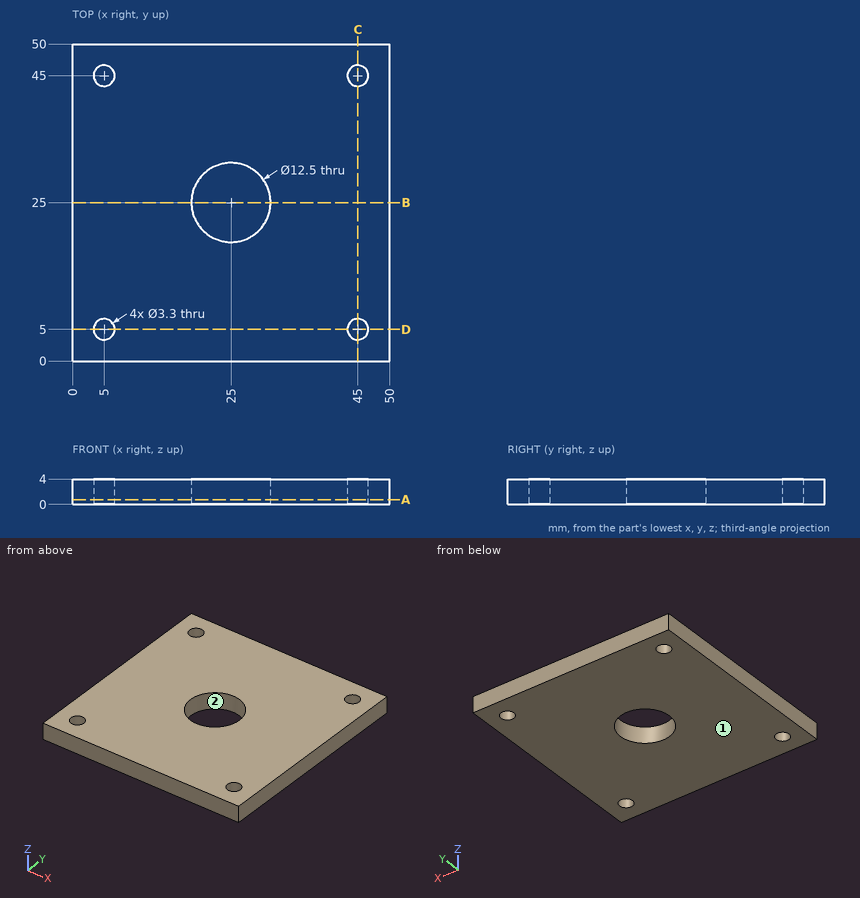
Input: dimensioned drawing with shaded views. Units: mm. Origin: part minimum x, y, z. Coordinates: 2 decimals unless noted, no trailing zeros. Loops run counter-clockwise (first coordinate to the right, second up) from the corner with the lowest first, then second, coordinate; pieces in that order, holes last. Notation, with made-up numbers: (22.25, 56.25) - (59.25, 56.25) arc R10 cw to (59.25, 65.25) - close; hole circle Ø1 at (53.5, 38.5). An arc over 180 degrees is marked (long way). One line per question, with ' | ' between items. Start each with the question number.
(1) Cut plane C-C on x = 45. Output: boundary loops of the cut face in (y, z).
(2) Cut plane A-A on z = 0.75. Output: boundary loops of the cut face in (x, y).
(3) Ray query, L1, parallel to Y at x = 5, z = 2.1; L2, parallel to Y at x = 25, z = 2.2; L3, parallel to X at y = 43.5, z = 2.8. Return the intervals inside material, ascending. Write a range as from..to.
(4) Cut plane B-B on y = 25. Output: boundary loops of the cut face in (x, z).
(5) Draft query along X for the marked faces 1 and 2. Return one class per face: +X half, -X half, draft (parallel to the pull), parting line (faces both ways), or undercut.
Here are the results:
1) outline: (0, 0) - (3.35, 0) - (3.35, 4) - (0, 4) - close; (6.65, 0) - (43.35, 0) - (43.35, 4) - (6.65, 4) - close; (46.65, 0) - (50, 0) - (50, 4) - (46.65, 4) - close
2) outline: (0, 0) - (50, 0) - (50, 50) - (0, 50) - close; hole circle Ø3.3 at (5, 5); hole circle Ø3.3 at (5, 45); hole circle Ø12.5 at (25, 25); hole circle Ø3.3 at (45, 5); hole circle Ø3.3 at (45, 45)
3) L1: 0..3.35, 6.65..43.35, 46.65..50 | L2: 0..18.75, 31.25..50 | L3: 0..4.31, 5.69..44.31, 45.69..50
4) outline: (0, 0) - (18.75, 0) - (18.75, 4) - (0, 4) - close; (31.25, 0) - (50, 0) - (50, 4) - (31.25, 4) - close
5) face 1: draft | face 2: undercut
